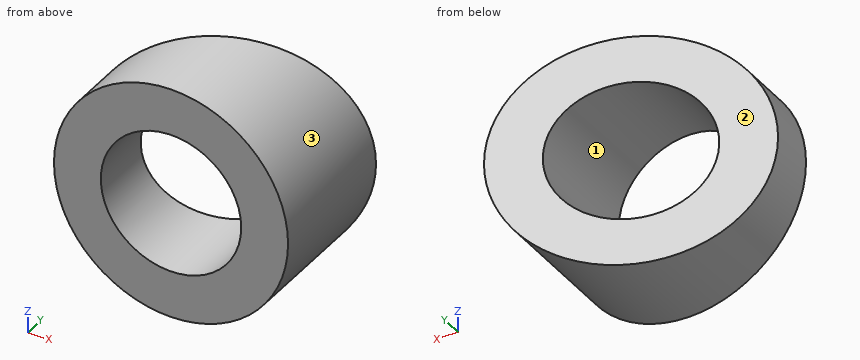
```python
from build123d import *

# Parameters (mm, degrees)
SKETCH_1_R          = 15
EXTRUDE_1_DEPTH     = 20
CUT_EXTRUDE_1_DEPTH = 16.5
SKETCH_7_R          = 9
CUT_EXTRUDE_2_DEPTH = 24.5


with BuildPart() as part:
    # 草图1 → 凸台-拉伸1 (new body)
    with BuildSketch(Plane(origin=(0, 0, 0), x_dir=(1, 0, 0), z_dir=(0, 1, 0))):
        Circle(SKETCH_1_R)
    extrude(amount=EXTRUDE_1_DEPTH)

    # 草图2 → 切除-拉伸1 (cut, symmetric)
    with BuildSketch(Plane.XY):
        Polygon((-15, 5.786796564), (15, 18.213203436), (15, 34.074049074), (-15, 34.074049074), align=None)
    extrude(amount=CUT_EXTRUDE_1_DEPTH, both=True, mode=Mode.SUBTRACT)

    # 草图7 → 切除-拉伸2 (cut)
    with BuildSketch(Plane.XZ):
        Circle(SKETCH_7_R)
    extrude(amount=-CUT_EXTRUDE_2_DEPTH, mode=Mode.SUBTRACT)


solid = part.part
```
The model under review builds one solid part; all positions refer to its coordinate system, in mm. Face numbers are marked on the shaded views. Round coordinates to 2 decimals unless told otherwise and drop trailing zeros. Write each loop counter-clockwise with the first axis right and the second up, starting at its lowest first coordinate (ties: lowest second). Pieces come first, ordered by that corner, then holes. Notation, with made-up numbers: (46.25, 19) - (89.25, 19) arc R12 cw to (89.25, 30) - close; hole circle Ø9 at (58.25, 87.5). An arc over 180 degrees is marked (long way). Answer as CSV lines item,"result". Start each with the question number.
(1) We need section B-B on z = 0.5. State the section outline as (x, y) points.
(2) For pin 1 Ø1 at (x, z) = (-4, 10.5) entering from +Y; pin 2 Ø3 at (y, z) = (15.5, -11.5) entering from +X; pin 3 Ø1.5 at (x, y) = (-4, 7) entering from -Z, all flat-tipped, find the tip position at first contact; note any pin that passes through.
(3) Draft analysis for pull direction Z (two halves, no side actions). For the marked faces 1, 2 and 3, state which applies: pulls with the +Z half, pulls with the -Z half, needs draft (parallel to the pull), parting line crosses it, or undercut.
(4) To check wall thickness, follow line 1 (Z direction, x = 0, y = 11); line 2 (X direction, y = 11, z = 0); line 3 (X direction, y = 6.5, z = -5.75). State the ranges of each line that lie inside material, in increasing order.
(5) We need section A-A on x = 1. State the section outline as (y, z) points, plus the area to 3 significant figures.
(6) We need section D-D on x = -12. State the section outline as (y, z) points, plus the area to 3 significant figures.
(7) We need section C-C on y = 4. State the section outline as (x, z) points, plus the area to 3 significant figures.
Worked answers:
1,outline,"(-14.99, 0) - (-8.99, 0) - (-8.99, 8.28) - (-14.99, 5.79) - close; (8.99, 0) - (14.99, 0) - (14.99, 18.21) - (8.99, 15.72) - close"
2,pin 1,"y = 10.55"
2,pin 2,"x = 11.18"
2,pin 3,"z = -14.64"
3,face 1,"undercut"
3,face 2,"needs draft"
3,face 3,"parting line crosses it"
4,line 1,"-15 to -9, 9 to 15"
4,line 2,"9 to 15"
4,line 3,"-13.28 to -6.92, 6.92 to 13.85"
5,outline,"(0, -14.97) - (12.41, -14.97) - (12.41, -8.94) - (0, -8.94) - close; (0, 8.94) - (12.41, 8.94) - (12.41, 14.97) - (0, 14.97) - close"
5,area,"150 mm²"
6,outline,"(0, -9) - (7.03, -9) - (7.03, 9) - (0, 9) - close"
6,area,"127 mm²"
7,outline,"circle Ø30 at (0, 0); hole circle Ø18 at (0, 0)"
7,area,"452 mm²"
